```python
from build123d import *

# Parameters (mm, degrees)
F0_W     = 38.1
F0_H     = 57.15
F1_DEPTH = 25.4
F3_DEPTH = 38.101
F4_W     = 19.05
F4_H     = 19.05
F5_DEPTH = 9.525


with BuildPart() as f1:
    # F0 (on Top) → F1 (new body)
    with BuildSketch(Plane.XY):
        with Locations((19.05, 28.575)):
            Rectangle(F0_W, F0_H)
    extrude(amount=F1_DEPTH)

    # F2 (on face) → F3 (cut, through all)
    with BuildSketch(Plane.YZ.offset(38.1)):
        Polygon((57.15, 25.4), (19.05, 25.4), (19.05, 19.05), (38.1, 19.05), (38.1, 9.525), (57.15, 9.525), align=None)
    extrude(amount=-F3_DEPTH, mode=Mode.SUBTRACT)

    # F4 (on face) → F5 (cut)
    with BuildSketch(Plane.XY.offset(19.05)):
        with Locations((19.05, 28.575)):
            Rectangle(F4_W, F4_H)
    extrude(amount=-F5_DEPTH, mode=Mode.SUBTRACT)


solid = f1.part
```
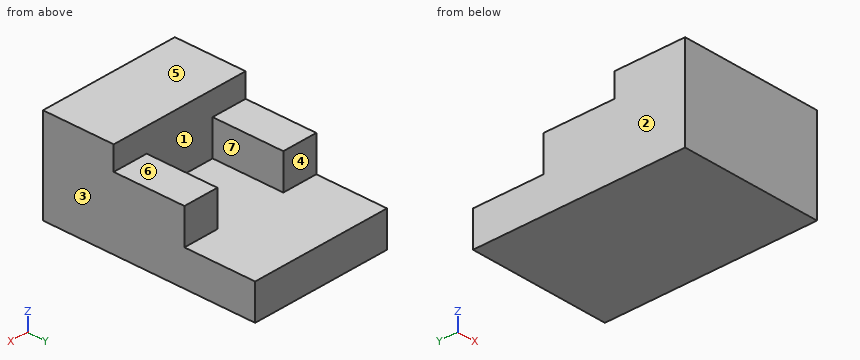
Could you check a few things on this model? Use its own coordinates, in mm. Face numbers are marked on the shaded views. A direction names the side the tool comes from. Coordinates: 2 decimals unless noted, no trailing zeros. Loops run counter-clockwise (first coordinate to the right, second up) from the corner with the lowest first, then second, coordinate; pieces in that order, holes last.
1) Will these pins go through, and if not, where does the flat tip stop? pin 1 Ø12 at (y, z) = (27.5, 16.5) entering from -X; pin 2 Ø3 at (x, y) = (35, 31.5) entering from +Z; pin 3 Ø5 at (x, z) = (18.5, 18) entering from +Y; pin 4 Ø5 at (x, z) = (5, 12.5) entering from +Y.
Reported:
pin 1: stops at x = 0
pin 2: stops at z = 19.05
pin 3: stops at y = 19.05
pin 4: stops at y = 38.1
2) Imagine slicing it at B-B (y = 25). List the corners of the cut face in (x, z) for me (3 decimals).
Reported:
outline: (0, 0) - (38.1, 0) - (38.1, 19.05) - (28.575, 19.05) - (28.575, 9.525) - (9.525, 9.525) - (9.525, 19.05) - (0, 19.05) - close
3) Which directions (+Z, -Z, +X, -X, +Y, -Y) give clear straight access to the entire face, cutting with the end or side of a thin tool? Please do the marked faces 5, 6 and 7.
Reported:
face 5: +Z, +X, -X, +Y, -Y
face 6: +Z, +X, -X, +Y
face 7: +Z, +Y
4) Imagine slicing it at D-D (z = 20.25). List the corners of the cut face in (x, y) for me, and give its area (3 significant figures).
Reported:
outline: (0, 0) - (38.1, 0) - (38.1, 19.05) - (0, 19.05) - close
area: 726 mm2
5) Imagine slicing it at C-C (x = 15.5). List the corners of the cut face in (y, z) for me (3 decimals).
Reported:
outline: (0, 0) - (57.15, 0) - (57.15, 9.525) - (19.05, 9.525) - (19.05, 25.4) - (0, 25.4) - close
6) Thinking about a two-plate mould opening in X: for the marked faces 1, 2, 3 and 4, which applies, released by +X, released by -X, zero draft, split by the parting line, or undercut?
Reported:
face 1: undercut
face 2: released by -X
face 3: released by +X
face 4: zero draft
7) Imagine slicing it at A-A (z = 13.5). List the corners of the cut face in (x, y) for me (3 decimals), and give its area (3 significant figures).
Reported:
outline: (0, 0) - (38.1, 0) - (38.1, 38.1) - (28.575, 38.1) - (28.575, 19.05) - (9.525, 19.05) - (9.525, 38.1) - (0, 38.1) - close
area: 1,090 mm2
8) Please list where these lines run through material, in increasing order: line 1 along X through (y, z) = (20.5, 10.5) (3 decimals); line 2 along Y through (x, z) = (29.5, 18); line 3 along Y through (x, z) = (28.5, 23.25).
Reported:
line 1: x = 0 to 9.525, 28.575 to 38.1
line 2: y = 0 to 38.1
line 3: y = 0 to 19.05
